Design review of the part built by this model. Coordinates are the model's own, in mm. Face numbers are marked on the shaded views. A direction names the side the tool comes from. Coordinates: 2 decimals unless noted, no trailing zeros. Loops run counter-clockwise (first coordinate to the right, second up) from the corner with the lowest first, then second, coordinate; pieces in that order, holes last. Notation, with made-up numbers: M 65.25,27.5 L 121.25,27.5 A18 ccw 121.25,36.5 Z; hole C 61.5,-36.75 d8. An arc over 180 degrees is marked long. Put each result on its own line as item: value. Start each with the question number.
(1) Take a section at D-D, the plane z = 1.25. Give the boundary of the cut face in (x, y), then the cut area to 3 significant figures.
(2) For probe 1 along Z at (x, y) = (-1, 1.45); probe 2 along Z at (x, y) = (-3, 0.15), list the stretches that pass through material, from the lowest coordinate up. Write a range as [from, to].
(3) For the marked faces 1, 2, 3 and 4, list the 3-axis set-ups (+Z, -Z, +X, -X, +Y, -Y) from which the entire face can be reached by the end or side of a thin tool; tool diameter is ignored.
(4) Take a section at C-C, the plane y = 0. Give the boundary of the cut face in (x, z).
(5) Take a section at A-A, the plane z = 0. Give the boundary of the cut face in (x, y), then the cut area to 3 significant figures.
(6) Take a section at B-B, the plane x = 0. Give the boundary of the cut face in (y, z), then the cut area to 3 significant figures.
```python
from build123d import *

# Parameters (mm, degrees)
SKETCH1_R           = 1.1
BOSS_EXTRUDE1_DEPTH = 3.6
CIRPATTERN1_COUNT   = 4
SKETCH3_W           = 4.8
SKETCH3_H           = 4.8
SKETCH3_W_2         = 2.2
SKETCH3_H_2         = 2.2
BOSS_EXTRUDE2_DEPTH = 1.5


with BuildPart() as part:
    # Sketch1 → Boss-Extrude1 (new, symmetric)
    with BuildSketch(Plane.XY):
        Circle(SKETCH1_R)
    boss_extrude1 = extrude(amount=BOSS_EXTRUDE1_DEPTH, both=True)

    # CirPattern1: Boss-Extrude1 ×4 about axis
    cirpattern1_axis = Axis((0, -1.485, 0), (0, 1, 0))
    for i in range(1, CIRPATTERN1_COUNT):
        add(boss_extrude1.rotate(cirpattern1_axis, i * 360 / CIRPATTERN1_COUNT))

    # Sketch3 → Boss-Extrude2 (add, symmetric)
    with BuildSketch(Plane(origin=(0, 0, 0), x_dir=(1, 0, 0), z_dir=(0, 1, 0))):
        Rectangle(SKETCH3_W, SKETCH3_H)
        Rectangle(SKETCH3_W_2, SKETCH3_H_2, mode=Mode.SUBTRACT)
        Rectangle(SKETCH3_W_2, SKETCH3_H_2)
    extrude(amount=BOSS_EXTRUDE2_DEPTH, both=True)


solid = part.part
```
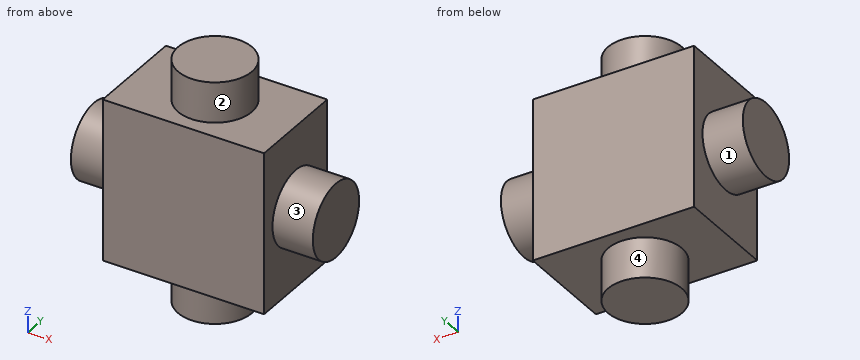
Computed values:
1. outline: M -2.4,-1.5 L 2.4,-1.5 L 2.4,1.5 L -2.4,1.5 Z
1. area: 14.4 mm^2
2. probe 1: z = [-2.4, 2.4]
2. probe 2: z = [-1.09, 1.09]
3. face 1: -X
3. face 2: +Z
3. face 3: +X
3. face 4: -Z
4. outline: M -3.6,-1.1 L -2.4,-1.1 L -2.4,-2.4 L -1.1,-2.4 L -1.1,-3.6 L 1.1,-3.6 L 1.1,-2.4 L 2.4,-2.4 L 2.4,-1.1 L 3.6,-1.1 L 3.6,1.1 L 2.4,1.1 L 2.4,2.4 L 1.1,2.4 L 1.1,3.6 L -1.1,3.6 L -1.1,2.4 L -2.4,2.4 L -2.4,1.1 L -3.6,1.1 Z
5. outline: M -3.6,-1.1 L -2.4,-1.1 L -2.4,-1.5 L 2.4,-1.5 L 2.4,-1.1 L 3.6,-1.1 L 3.6,1.1 L 2.4,1.1 L 2.4,1.5 L -2.4,1.5 L -2.4,1.1 L -3.6,1.1 Z
5. area: 19.7 mm^2
6. outline: M -1.5,-2.4 L -1.1,-2.4 L -1.1,-3.6 L 1.1,-3.6 L 1.1,-2.4 L 1.5,-2.4 L 1.5,2.4 L 1.1,2.4 L 1.1,3.6 L -1.1,3.6 L -1.1,2.4 L -1.5,2.4 Z
6. area: 19.7 mm^2
